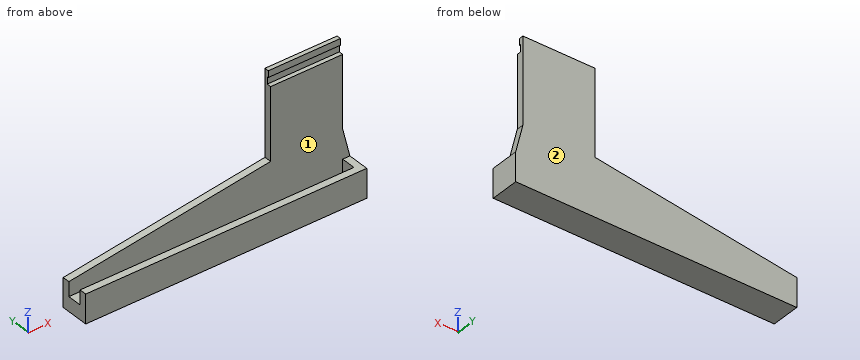
from build123d import *

# Parameters (mm, degrees)
F0_W      = 190
F0_H      = 5
F1_DEPTH  = 20
F2_W      = 190
F2_H      = 10
F3_DEPTH  = 10
F4_W      = 50
F4_H      = 5
F5_DEPTH  = 70
F7_DEPTH  = 5
F8_W      = 50
F8_H      = 2
F9_DEPTH  = 5
F10_W     = 50
F10_H     = 3
F11_DEPTH = 4.5


with BuildPart() as f1:
    # F0 (on Top) → F1 (new body)
    with BuildSketch(Plane.XY):
        with Locations((95, 2.5)):
            Rectangle(F0_W, F0_H)
        Polygon((190, 5), (190, 0), (195, 0), (195, 20), (190, 20), (190, 15), align=None)
        with Locations((95, 17.5)):
            Rectangle(F0_W, F0_H)
    extrude(amount=F1_DEPTH)

    # F2 (on Top) → F3 (join)
    with BuildSketch(Plane.XY):
        with Locations((95, 10)):
            Rectangle(F2_W, F2_H)
    extrude(amount=F3_DEPTH)

    # F4 (on face) → F5 (join)
    with BuildSketch(Plane.XY.offset(20)):
        with Locations((165, 17.5)):
            Rectangle(F4_W, F4_H)
    extrude(amount=F5_DEPTH)

    # F6 (on face) → F7 (join)
    with BuildSketch(Plane(origin=(0, 20, 0), x_dir=(-1, 0, 0), z_dir=(0, 1, 0))):
        Polygon((-190, 40), (-195, 20), (-190, 20), align=None)
        Polygon((-140, 40), (-140, 20), (0, 20), align=None)
    extrude(amount=-F7_DEPTH)

    # F8 (on face) → F9 (join)
    with BuildSketch(Plane.XY.offset(90)):
        with Locations((165, 19)):
            Rectangle(F8_W, F8_H)
    extrude(amount=F9_DEPTH)

    # F10 (on face) → F11 (join)
    with BuildSketch(Plane.XY.offset(95)):
        with Locations((165, 18.5)):
            Rectangle(F10_W, F10_H)
    extrude(amount=F11_DEPTH)


solid = f1.part
Verification items for the finished model (mm, model axes). Face numbers are marked on the shaded views. A direction names the side the tool comes from. Coordinates: 2 decimals unless noted, no trailing zeros. Order: outer loops, then holes, each group sorted by start corner. A loop starts at its lowest first (then second) coordinate and runs counter-clockwise, first axis right, second up. Notation, with made-up numbers: (7, 49.5) -> (54, 49.5) arc R20 ccw to (54, 69.5) -> close; hole circle Ø10 at (0, -25.75). An arc over 180 degrees is marked (long way). Put each result on its own line as item: value. Start each with the question number.
1. Access from +Z, -Z, +X, -X, +Y, -Y to the whole of each face (thin tool, end or side, straight path). Record for the marked faces 1 and 2.
2. Cross-section at D-D, the plane x = 40.5. Record the boundary of the cut face in (y, z), then the cut area to 3 significant figures.
3. Material ranges on L1, parallel to Y at x = 130.5, z = 11; L2, parallel to Y at x = 158, z = 72; L3, parallel to Z at x = 177, y = 4.75, recorded low to high. Write a range as [from, to].
4. Go/stop test with flat-tipped pins: pin 1 Ø2.5 at (y, z) = (18.5, 59.5) entering from +X; pin 2 Ø5.5 at (x, z) = (170.5, 92.5) entering from -Y; pin 3 Ø6 at (y, z) = (17.5, 45.5) entering from -X. Record where each tip stops, or that it passes through.
5. Cross-section at A-A, the plane x = 178.5. Record the boundary of the cut face in (y, z), then the cut area to 4 significant figures.
6. Cross-section at C-C, the plane z = 12. Record the boundary of the cut face in (x, y).
7. Cross-section at B-B, the plane y = 10.75. Record the boundary of the cut face in (x, z).
Computed:
1. face 1: +Z, -X
1. face 2: +Z, -Z, +X, -X, +Y
2. outline: (0, 0) -> (20, 0) -> (20, 25.79) -> (15, 25.79) -> (15, 10) -> (5, 10) -> (5, 20) -> (0, 20) -> close
2. area: 329 mm2
3. L1: [0, 5], [15, 20]
3. L2: [15, 20]
3. L3: [0, 20]
4. pin 1: x = 190
4. pin 2: y = 15
4. pin 3: x = 140
5. outline: (0, 0) -> (20, 0) -> (20, 99.5) -> (17, 99.5) -> (17, 95) -> (18, 95) -> (18, 90) -> (15, 90) -> (15, 10) -> (5, 10) -> (5, 20) -> (0, 20) -> close
5. area: 673.5 mm2
6. outline: (0, 0) -> (195, 0) -> (195, 20) -> (0, 20) -> (0, 15) -> (190, 15) -> (190, 5) -> (0, 5) -> close
7. outline: (0, 0) -> (195, 0) -> (195, 20) -> (190, 20) -> (190, 10) -> (0, 10) -> close
